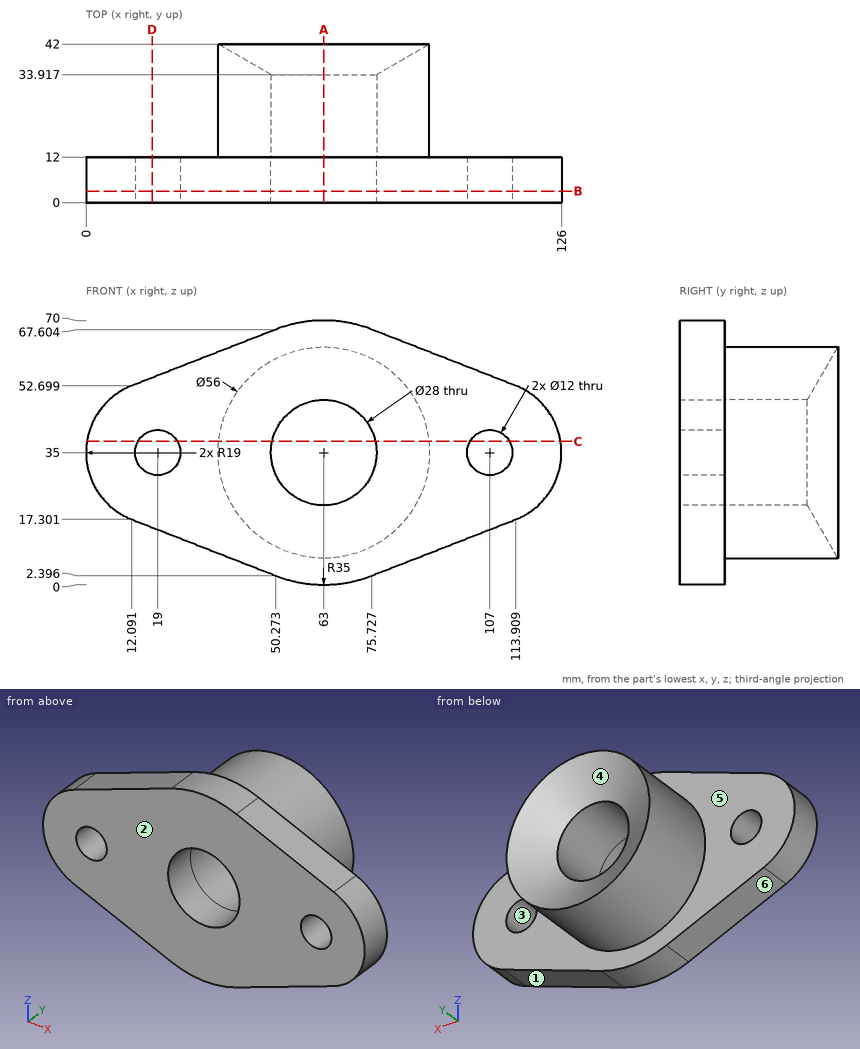
Can you work these out from the drawing? Everything is in mm from the part's minimum corner. A direction names the side the tool comes from. Give positions to 0.01 mm unless a question says otherwise; leave off trailing zeros. Loops run counter-clockwise (first coordinate to the right, second up) from the corner with the lowest first, then second, coordinate; pieces in that order, holes last. Notation, with made-up numbers: (38, 46.5) -> (53, 46.5) arc R28 cw to (53, 74.5) -> close; hole circle Ø1 at (27, 49). An arc over 180 degrees is marked (long way). Put each result on its own line as item: value.
(1) Imagine slicing it at D-D on x = 17.5. Write out the boundary of the cut face in (y, z).
Computed:
outline: (0, 15.19) -> (12, 15.19) -> (12, 29.19) -> (0, 29.19) -> close; (0, 40.81) -> (12, 40.81) -> (12, 54.81) -> (0, 54.81) -> close
(2) Imagine slicing it at C-C on z = 38. State how many separate pieces and enclosed holes the cut face has, plus the area to 3 significant figures.
Computed:
separate pieces: 4
enclosed holes: 0
area: 1,660 mm^2
(3) Thinking about a two-plate mould opening in Z: for the marked faces 1, 2, 3 and 4, which applies, pulls with the +Z half, pulls with the -Z half, needs draft (parallel to the pull), parting line crosses it, or undercut?
Computed:
face 1: pulls with the -Z half
face 2: needs draft
face 3: undercut
face 4: undercut
(4) Please list where these lines run through material, in increasing order: probe 1 along X at (y, z) = (20.25, 35); probe 2 along X at (y, z) = (14, 36.5); probe 3 along Z at (x, y) = (73, 37) (1 decimal). Write a range as [from, to].
Computed:
probe 1: [35, 49], [77, 91]
probe 2: [35.04, 49.08], [76.92, 90.96]
probe 3: [8.8, 18.4], [51.6, 61.2]
(5) Imagine slicing it at B-B on y = 3. Write out the boundary of the cut face in (x, z), plus the area to 3 significant figures.
Computed:
outline: (12.09, 17.3) -> (50.27, 2.4) arc R35 ccw to (75.73, 2.4) -> (113.91, 17.3) arc R19 ccw to (113.91, 52.7) -> (75.73, 67.6) arc R35 ccw to (50.27, 67.6) -> (12.09, 52.7) arc R19 ccw to start; hole circle Ø12 at (19, 35); hole circle Ø28 at (63, 35); hole circle Ø12 at (107, 35)
area: 5,360 mm^2
(6) I'm going to push flat-ended pins straight in: pin 1 Ø1 at (y, z) = (22, 57) entering from -X; pin 2 Ø1.5 at (x, z) = (22.5, 45.5) entering from +Y; pin 3 Ø9.5 at (x, z) = (107, 35) entering from -Y; pin 4 Ø10 at (x, y) = (61.5, 18.5) entering from +Z. Where does each tip first touch, or does it pass through?
Computed:
pin 1: x = 45.06
pin 2: y = 12
pin 3: through
pin 4: z = 63
(7) For the marked faces 5 and 6, which set-ups out of +Z, -Z, +X, -X, +Y, -Y let a thin tool reach every point of the face, with its end or its side?
Computed:
face 5: +Y
face 6: -Z, -X, +Y, -Y
(8) Imagine slicing it at A-A on x = 63. Write out the boundary of the cut face in (y, z).
Computed:
outline: (0, 0) -> (12, 0) -> (12, 7) -> (42, 7) -> (33.92, 21) -> (0, 21) -> close; (0, 49) -> (33.92, 49) -> (42, 63) -> (12, 63) -> (12, 70) -> (0, 70) -> close
